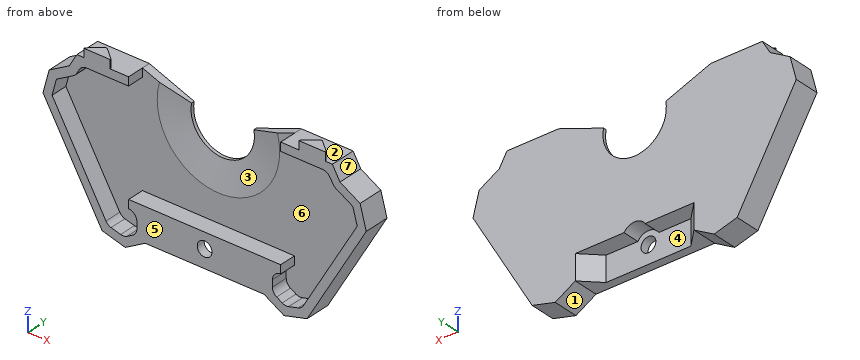
from build123d import *

# Parameters (mm, degrees)
BOSS_EXTRUDE6_DEPTH   = 2
BOSS_EXTRUDE6_2_DEPTH = 2
BOSS_EXTRUDE7_DEPTH   = 4
SKETCH15_W            = 28.094808214
SKETCH15_H            = 7.894882233
SKETCH15_R            = 1.75
BOSS_EXTRUDE8_DEPTH   = 2
BOSS_EXTRUDE9_DEPTH   = 2
FILLET3_R             = 0.5
FILLET3_OF_MIRROR2_R  = 0.5
BOSS_EXTRUDE10_DEPTH  = 2
BOSS_EXTRUDE11_DEPTH  = 4
CHAMFER2_SIZE         = 4
FILLET4_R             = 2
CHAMFER3_SIZE         = 7
CHAMFER3_SIZE2        = 1.234288865


# Some blends are built 0.0001 mm under size
with BuildPart() as part:
    # Sketch13 → Boss-Extrude6 (new body)
    with BuildSketch(Plane(origin=(0, 0, 0), x_dir=(1, 0, 0), z_dir=(0, 1, 0))):
        Polygon((-18, 21), (-14.047404107, 21), (-14.047404107, 28.894882233), (-18.803847577, 31.641016151), (-24.267949192, 30.176914536), (-38.267949192, 5.92820323), (-36.803847577, 0.464101615), (-32.047404107, -2.282032303), (-30.244289874, -5.405117767), (-30.12881982, -5.405117767), (-20, -5.405117767), (-18, -5.405117767), align=None)
    extrude(amount=BOSS_EXTRUDE6_DEPTH)



with BuildPart() as body_2:
    # Sketch13 → Boss-Extrude6 2 (new body)
    with BuildSketch(Plane(origin=(0, 0, 0), x_dir=(1, 0, 0), z_dir=(0, 1, 0))):
        Polygon((18, -5.405117767), (18, 21), (14.047404107, 21), (14.047404107, 28.894882233), (18.803847577, 31.641016151), (24.267949192, 30.176914536), (38.267949192, 5.92820323), (36.803847577, 0.464101615), (32.047404107, -2.282032303), (30.244289874, -5.405117767), (30.12881982, -5.405117767), (26.664718205, -5.405117767), (20, -5.405117767), align=None)
    extrude(amount=BOSS_EXTRUDE6_2_DEPTH)


with BuildPart() as part_1:
    add(part.part)

    add(body_2.part)  # Boss-Extrude7 merges body 2
    # Sketch14 → Boss-Extrude7 (add)
    with BuildSketch(Plane.XZ):
        Polygon((-30.244289874, 5.405117767), (-18, 5.405117767), (-18, 3.405117767), (-29.089589336, 3.405117767), (-30.583302492, 0.817930688), (-35.086408642, -1.78193886), (-36.121684822, -5.645642165), (-22.950111947, -28.459475601), (-19.086408642, -29.494751781), (-16.047404107, -27.740181695), (-16.047404107, -23), (-18, -23), (-18, -21), (-14.047404107, -21), (-14.047404107, -28.894882233), (-18.803847577, -31.641016151), (-24.267949192, -30.176914536), (-38.267949192, -5.92820323), (-36.803847577, -0.464101615), (-32.047404107, 2.282032303), align=None)
        Polygon((14.047404107, -21), (18, -21), (18, -23), (16.047404107, -23), (16.047404107, -27.740181695), (19.086408642, -29.494751781), (22.950111947, -28.459475601), (36.121684822, -5.645642165), (35.086408642, -1.78193886), (30.583302492, 0.817930688), (29.089589336, 3.405117767), (18, 3.405117767), (18, 5.405117767), (30.244289874, 5.405117767), (32.047404107, 2.282032303), (36.803847577, -0.464101615), (38.267949192, -5.92820323), (24.267949192, -30.176914536), (18.803847577, -31.641016151), (14.047404107, -28.894882233), align=None)
    extrude(amount=BOSS_EXTRUDE7_DEPTH)

    # Sketch15 → Boss-Extrude8 (add)
    with BuildSketch(Plane.XZ.offset(4)):
        with Locations((0, -24.947441117)):
            Rectangle(SKETCH15_W, SKETCH15_H)
        with Locations(Location((0, -24.644882233, 0), (0, 0, 270))):
            Circle(SKETCH15_R, mode=Mode.SUBTRACT)
    extrude(amount=-BOSS_EXTRUDE8_DEPTH)

    # Sketch16 → Boss-Extrude9 (add)
    with BuildSketch(Plane.XY.offset(5.405117767)):
        Polygon((-28.574119282, -3.76), (-28.574119282, -4), (-22.4, -4), (-22.4, -3.76), (-25.487059641, -1.104129474), align=None)
    boss_extrude9 = extrude(amount=BOSS_EXTRUDE9_DEPTH)

    # Fillet3
    fillet3_edges = [part_1.edges().sort_by_distance(p)[0] for p in [
        (-25.487059641, -1.104129474, 6.405117767),
    ]]
    fillet(fillet3_edges, radius=FILLET3_R)

    # Mirror2: Boss-Extrude9 across plane
    add(boss_extrude9.mirror(Plane(origin=(0, 0, 0), x_dir=(0, 0, 1), z_dir=(1, 0, 0))))

    # Fillet3 of Mirror2
    fillet3_of_mirror2_edges = [part_1.edges().sort_by_distance(p)[0] for p in [
        (25.487059641, -1.104129474, 6.405117767),
    ]]
    fillet(fillet3_of_mirror2_edges, radius=FILLET3_OF_MIRROR2_R)

    # Sketch17 → Boss-Extrude10 (add)
    with BuildSketch(Plane(origin=(0, 2, 0), x_dir=(1, 0, 0), z_dir=(0, 1, 0))):
        with BuildLine():
            Line((-18, -5.405117767), (-7.367200558, -1.405117767))
            ThreePointArc((-7.367200558, -1.405117767), (0, 7.5), (7.367200558, -1.405117767))
            Line((7.367200558, -1.405117767), (18, -5.405117767))
            Line((18, -5.405117767), (18, 21))
            Line((18, 21), (-18, 21))
            Line((-18, 21), (-18, -5.405117767))
        make_face()
    extrude(amount=-BOSS_EXTRUDE10_DEPTH)

    # Sketch18 → Boss-Extrude11 (add)
    with BuildSketch(Plane(origin=(0, -2, 0), x_dir=(1, 0, 0), z_dir=(0, 1, 0))):
        with BuildLine():
            Line((14.047404107, 21), (-14.047404107, 21))
            Line((-14.047404107, 21), (-14.047404107, 23))
            Line((-14.047404107, 23), (-2.508856799, 23))
            ThreePointArc((-2.508856799, 23), (0, 21.644882233), (2.508856799, 23))
            Line((2.508856799, 23), (14.047404107, 23))
            Line((14.047404107, 23), (14.047404107, 21))
        make_face()
    extrude(amount=BOSS_EXTRUDE11_DEPTH)

    # Chamfer2
    chamfer2_edges = [part_1.edges().sort_by_distance(p)[0] for p in [
        (14.047404107, -2, -25.947441117),
        (-14.047404107, -2, -25.947441117),
    ]]
    chamfer(chamfer2_edges, length=CHAMFER2_SIZE - 0.0001)  # a hair under: the kernel refuses the full size

    # Fillet4
    # the kernel refuses this fillet: 2 mm, written as the material it adds along each edge
    with BuildSketch(Plane(origin=(29.089589336, 2.886751346, 3.405117767), x_dir=(0.4999999999999999, 0, -0.8660254037844386), z_dir=(0, -1, 0))) as fillet4_piece_1_section:
        with BuildLine():
            CenterArc((FILLET4_R * 0.57735026919, -FILLET4_R), FILLET4_R, 90, 60)
            Line((-FILLET4_R * 0.288675134595, -FILLET4_R * 0.5), (0, 0))
            Line((0, 0), (FILLET4_R * 0.57735026919, 0))
        make_face()
    fillet4_piece_1 = extrude(amount=6.886751346, mode=Mode.PRIVATE)
    fillet4_piece_1 = split(fillet4_piece_1, bisect_by=Plane(origin=(28.968451808, 2, 3.195301414), z_dir=(0, -1, 0)), keep=Keep.TOP, mode=Mode.PRIVATE)
    add(fillet4_piece_1)
    with BuildSketch(Plane(origin=(-29.089589336, 2.886751346, 3.405117767), x_dir=(1, 0, 0), z_dir=(0, -1, 0))) as fillet4_piece_2_section:
        with BuildLine():
            CenterArc((FILLET4_R * 0.57735026919, -FILLET4_R), FILLET4_R, 90, 60)
            Line((-FILLET4_R * 0.288675134595, -FILLET4_R * 0.5), (0, 0))
            Line((0, 0), (FILLET4_R * 0.57735026919, 0))
        make_face()
    fillet4_piece_2 = extrude(amount=6.886751346, mode=Mode.PRIVATE)
    fillet4_piece_2 = split(fillet4_piece_2, bisect_by=Plane(origin=(-28.968451808, 2, 3.195301414), z_dir=(0, -1, 0)), keep=Keep.TOP, mode=Mode.PRIVATE)
    add(fillet4_piece_2)
    with BuildSketch(Plane(origin=(22.950111947, 2.071067812, -28.459475601), x_dir=(-0.9659258262890683, 0, -0.2588190451025206), z_dir=(0, -1, 0))) as fillet4_piece_3_section:
        with BuildLine():
            CenterArc((FILLET4_R * 0.414213562373, -FILLET4_R), FILLET4_R, 90, 45)
            Line((-FILLET4_R * 0.292893218813, -FILLET4_R * 0.292893218813), (0, 0))
            Line((0, 0), (FILLET4_R * 0.414213562373, 0))
        make_face()
    fillet4_piece_3 = extrude(amount=6.071067812, mode=Mode.PRIVATE)
    fillet4_piece_3 = split(fillet4_piece_3, bisect_by=Plane(origin=(22.870823982, 2, -28.356145514), z_dir=(0, -1, 0)), keep=Keep.TOP, mode=Mode.PRIVATE)
    add(fillet4_piece_3)
    with BuildSketch(Plane(origin=(19.086408642, 2.071067812, -29.494751781), x_dir=(-0.8660254037844382, 0, 0.500000000000001), z_dir=(0, -1, 0))) as fillet4_piece_4_section:
        with BuildLine():
            CenterArc((FILLET4_R * 0.414213562373, -FILLET4_R), FILLET4_R, 90, 45)
            Line((-FILLET4_R * 0.292893218813, -FILLET4_R * 0.292893218813), (0, 0))
            Line((0, 0), (FILLET4_R * 0.414213562373, 0))
        make_face()
    fillet4_piece_4 = extrude(amount=6.071067812, mode=Mode.PRIVATE)
    fillet4_piece_4 = split(fillet4_piece_4, bisect_by=Plane(origin=(19.10340899, 2, -29.365621318), z_dir=(0, -1, 0)), keep=Keep.TOP, mode=Mode.PRIVATE)
    add(fillet4_piece_4)
    with BuildSketch(Plane(origin=(16.047404107, 2.886751346, -27.740181695), x_dir=(0, 0, 1), z_dir=(0, -1, 0))) as fillet4_piece_5_section:
        with BuildLine():
            CenterArc((FILLET4_R * 0.57735026919, -FILLET4_R), FILLET4_R, 90, 60)
            Line((-FILLET4_R * 0.288675134595, -FILLET4_R * 0.5), (0, 0))
            Line((0, 0), (FILLET4_R * 0.57735026919, 0))
        make_face()
    fillet4_piece_5 = extrude(amount=6.886751346, mode=Mode.PRIVATE)
    fillet4_piece_5 = split(fillet4_piece_5, bisect_by=Plane(origin=(16.257220459, 2, -27.619044168), z_dir=(0, -1, 0)), keep=Keep.TOP, mode=Mode.PRIVATE)
    add(fillet4_piece_5)
    with BuildSketch(Plane(origin=(-22.950111947, 2.071067812, -28.459475601), x_dir=(-0.500000000000001, 0, 0.8660254037844382), z_dir=(0, -1, 0))) as fillet4_piece_6_section:
        with BuildLine():
            CenterArc((FILLET4_R * 0.414213562373, -FILLET4_R), FILLET4_R, 90, 45)
            Line((-FILLET4_R * 0.292893218813, -FILLET4_R * 0.292893218813), (0, 0))
            Line((0, 0), (FILLET4_R * 0.414213562373, 0))
        make_face()
    fillet4_piece_6 = extrude(amount=6.071067812, mode=Mode.PRIVATE)
    fillet4_piece_6 = split(fillet4_piece_6, bisect_by=Plane(origin=(-22.870823982, 2, -28.356145514), z_dir=(0, -1, 0)), keep=Keep.TOP, mode=Mode.PRIVATE)
    add(fillet4_piece_6)
    with BuildSketch(Plane(origin=(-19.086408642, 2.071067812, -29.494751781), x_dir=(-0.9659258262890694, 0, 0.2588190451025166), z_dir=(0, -1, 0))) as fillet4_piece_7_section:
        with BuildLine():
            CenterArc((FILLET4_R * 0.414213562373, -FILLET4_R), FILLET4_R, 90, 45)
            Line((-FILLET4_R * 0.292893218813, -FILLET4_R * 0.292893218813), (0, 0))
            Line((0, 0), (FILLET4_R * 0.414213562373, 0))
        make_face()
    fillet4_piece_7 = extrude(amount=6.071067812, mode=Mode.PRIVATE)
    fillet4_piece_7 = split(fillet4_piece_7, bisect_by=Plane(origin=(-19.10340899, 2, -29.365621318), z_dir=(0, -1, 0)), keep=Keep.TOP, mode=Mode.PRIVATE)
    add(fillet4_piece_7)
    with BuildSketch(Plane(origin=(-16.047404107, 2.886751346, -27.740181695), x_dir=(-0.8660254037844385, 0, -0.5000000000000003), z_dir=(0, -1, 0))) as fillet4_piece_8_section:
        with BuildLine():
            CenterArc((FILLET4_R * 0.57735026919, -FILLET4_R), FILLET4_R, 90, 60)
            Line((-FILLET4_R * 0.288675134595, -FILLET4_R * 0.5), (0, 0))
            Line((0, 0), (FILLET4_R * 0.57735026919, 0))
        make_face()
    fillet4_piece_8 = extrude(amount=6.886751346, mode=Mode.PRIVATE)
    fillet4_piece_8 = split(fillet4_piece_8, bisect_by=Plane(origin=(-16.257220459, 2, -27.619044168), z_dir=(0, -1, 0)), keep=Keep.TOP, mode=Mode.PRIVATE)
    add(fillet4_piece_8)
    with BuildSketch(Plane(origin=(-16.047404107, 5, -23), x_dir=(0, 0, -1), z_dir=(0, -1, 0))) as fillet4_piece_9_section:
        with BuildLine():
            CenterArc((FILLET4_R, -FILLET4_R), FILLET4_R, 90, 90)
            Line((0, -FILLET4_R), (0, 0))
            Line((0, 0), (FILLET4_R, 0))
        make_face()
    fillet4_piece_9 = extrude(amount=9, mode=Mode.PRIVATE)
    fillet4_piece_9 = split(fillet4_piece_9, bisect_by=Plane(origin=(-18, -2, -23.446740496), z_dir=(1, 0, 0)), keep=Keep.TOP, mode=Mode.PRIVATE)
    fillet4_piece_9 = split(fillet4_piece_9, bisect_by=Plane(origin=(-16.494124288, 2, -23.446740496), z_dir=(0, -1, 0)), keep=Keep.TOP, mode=Mode.PRIVATE)
    add(fillet4_piece_9)
    with BuildSketch(Plane(origin=(16.047404107, 5, -23), x_dir=(1, 0, 0), z_dir=(0, -1, 0))) as fillet4_piece_10_section:
        with BuildLine():
            CenterArc((FILLET4_R, -FILLET4_R), FILLET4_R, 90, 90)
            Line((0, -FILLET4_R), (0, 0))
            Line((0, 0), (FILLET4_R, 0))
        make_face()
    fillet4_piece_10 = extrude(amount=9, mode=Mode.PRIVATE)
    fillet4_piece_10 = split(fillet4_piece_10, bisect_by=Plane(origin=(18, -2, -23.446740496), z_dir=(-1, 0, 0)), keep=Keep.TOP, mode=Mode.PRIVATE)
    fillet4_piece_10 = split(fillet4_piece_10, bisect_by=Plane(origin=(16.494124288, 2, -23.446740496), z_dir=(0, -1, 0)), keep=Keep.TOP, mode=Mode.PRIVATE)
    add(fillet4_piece_10)
    # the kernel refuses this fillet: 2 mm, written as the material it takes off along each edge
    with BuildSketch(Plane(origin=(30.583302492, 0, 0.817930688), x_dir=(0.8660254037844376, 0, -0.500000000000002), z_dir=(0, -1, 0)), Plane(origin=(-30.583302492, 0, 0.817930688), x_dir=(0.5000000000000039, 0, 0.8660254037844364), z_dir=(0, -1, 0))) as fillet4_2_piece_1:
        with BuildLine():
            CenterArc((FILLET4_R * 0.267949192431, FILLET4_R), FILLET4_R, 240, 30)
            Line((-FILLET4_R * 0.232050807569, FILLET4_R * 0.133974596216), (0, 0))
            Line((0, 0), (FILLET4_R * 0.267949192431, 0))
        make_face()
    extrude(amount=5.339745962, mode=Mode.SUBTRACT)

    # Chamfer3
    chamfer3_edges = [part_1.edges().sort_by_distance(p)[0] for p in [
        (0, 0, -7.5),
    ]]
    chamfer3_side = [part_1.faces().sort_by_distance(p)[0] for p in [
        (0, 0, -10.489967156),
    ]]
    chamfer(chamfer3_edges, length=CHAMFER3_SIZE, length2=CHAMFER3_SIZE2, reference=chamfer3_side[0])


solid = part_1.part
Here's how the part is built. I have some questions about the finished solid (model axes, mm). Face numbers are marked on the shaded views. A direction names the side the tool comes from. Coordinates: 2 decimals unless noted, no trailing zeros. Write each loop counter-clockwise with the first axis right and the second up, starting at its lowest first coordinate (ties: lowest second). Pieces come first, ordered by that corner, then holes.
Item 1: I want a section at A-A on x = 0. Write out the boundary of the cut face in (y, z).
Item 2: I want a section at B-B on x = 21. Write out the boundary of the cut face in (y, z), and give its area (3 significant figures).
Item 3: I want a section at C-C on x = 33. Write out the boundary of the cut face in (y, z), and give its area (3 significant figures).
Item 4: On a 3-axis mill with a long thin cutter (end or side, diameter ignored), from which of +Z, -Z, +X, -X, +Y, -Y can I reach the whole of each face in a straight line? I mean the marked faces 1, 2, 3 and 4. Say none if no direction works.
Item 5: If we mould it in two halves opening along X, with no side actions, what happens to the marked faces 5, 6 and 7? For each: +X half, -X half, draft (parallel to the pull), parting line (faces both ways), or undercut.
Item 6: If I drill on line 1 (X direction, y = -2.7, z = -25.5); line 2 (X direction, y = -2.8, z = -24.5); line 3 (Z direction, x = 0, y = 1.8), over which ranges is the centre line in solid material (lowest first)?
Item 7: Will these pins go through, and if not, where does the flat tip stop? pin 1 (0.8 mm diameter, centred on y = -2, z = -26, fed in from -X); pin 2 (3 mm diameter, centred on x = 9, y = 0, fed in from -Z); pin 3 (1.5 mm diameter, centred on x = -30, y = -2.5, fed in from +Z).
Findings below:
1. outline: (-4, -28.89) - (-2, -28.89) - (-2, -26.39) - (-4, -26.39) - close; (-4, -22.89) - (-2, -22.89) - (-2, -21.64) - (2, -21.64) - (2, -7.5) - (1.23, -7.5) - (0, -14.5) - (0, -21) - (-4, -21) - close
2. outline: (-4, -31.05) - (2, -31.05) - (2, 5.41) - (-4, 5.41) - (-4, 3.41) - (0, 3.41) - (0, -28.98) - (-4, -28.98) - close
2. area: 89.2 mm2
3. outline: (-4, -15.05) - (2, -15.05) - (2, 1.73) - (-4, 1.73) - (-4, -0.58) - (0, -0.58) - (0, -11.05) - (-4, -11.05) - close
3. area: 58.8 mm2
4. face 1: -Z, +Y, -Y
4. face 2: +Z, +Y
4. face 3: -Y
4. face 4: -Z, +Y
5. face 5: draft
5. face 6: undercut
5. face 7: +X half
6. line 1: x = -26.97 to -24.66, -16.05 to -1.53, 1.53 to 16.05, 24.66 to 26.97
6. line 2: x = -27.55 to -25.24, -16.11 to -1.74, 1.74 to 16.11, 25.24 to 27.55
6. line 3: z = -21.64 to -7.5
7. pin 1: stops at x = -26.91
7. pin 2: stops at z = -23
7. pin 3: stops at z = 5.41
